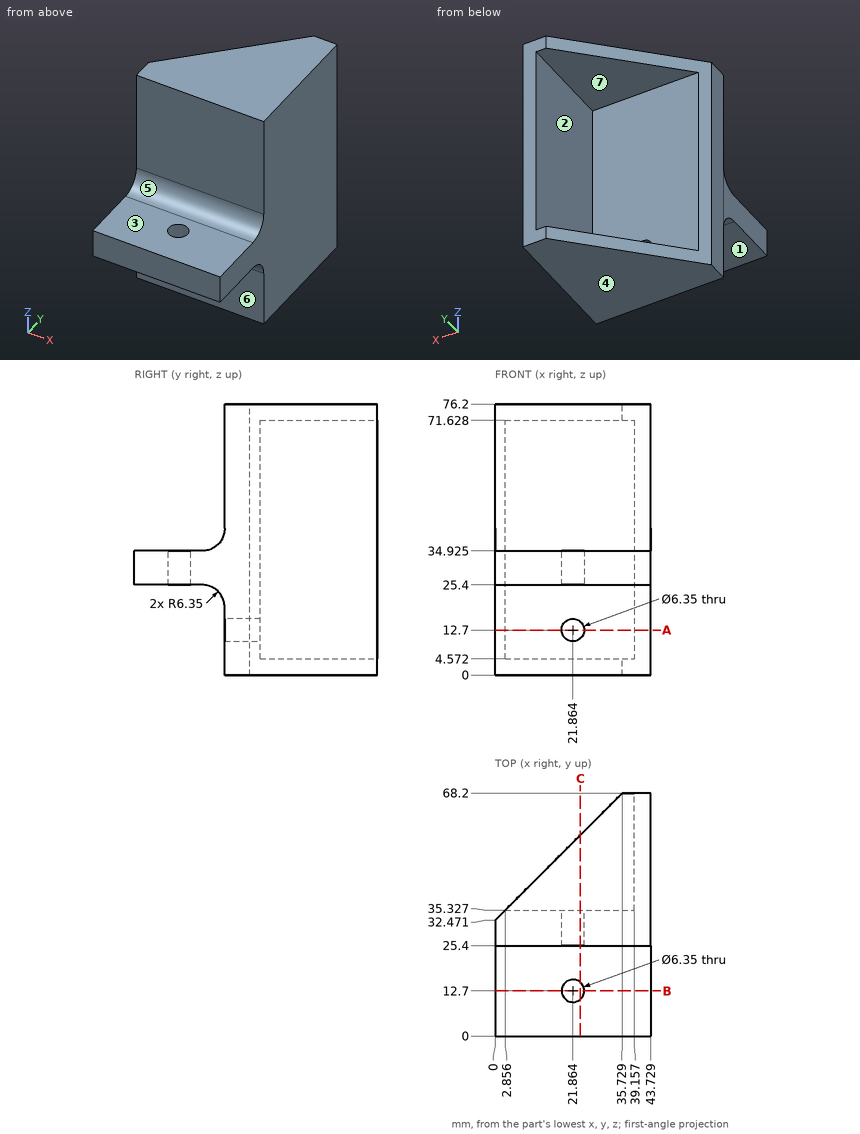
Geometry check sheet. Reference: drawing and pictorial views, mm from the part's lowest x, y, z. A direction names the side the tool comes from. Coordinates: 2 decimals unless noted, no trailing zeros. Order: outer loops, then holes, each group sorted by start corner. A loop starts at its lowest first (then second) coordinate and runs counter-clockwise, first axis right, second up.
Item 1: Tool access check on the marked faces 1, 2 and 3. Record the directions out of +Z, -Z, +X, -X, +Y, -Y that give a thin tool (end or side, any length) a straight path to the whole face; none if there is none.
Item 2: Section check A-A (z = 12.7). Enter the section's corners in (x, y).
Item 3: Depth check by flat-ended pin: pin 1 (17.5 mm diameter, centred on x = 32.5, z = 63, fed in from -Y); pin 2 (21 mm diameter, centred on x = 11, y = 10, fed in from -Z); pin 3 (5 mm diameter, centred on x = 29.5, z = 34, fed in from +Y). Enter the tip coordinate at first touch or a pass-through.
Item 4: Mould release check, pull along Z, two halves, no side actions. Record for the marked faces 4, 5, 6 and 7: released by +Z, released by -Z, zero draft, split by the parting line, or undercut.
Item 5: Scan lines: line 1 along Z through (x, y) = (17.5, 16) (1 decimal); line 2 along Y through (x, z) = (14, 19); line 3 along X through (y, z) = (12, 31). Record each from-to range of solid material in increasing order.
Item 6: Section check B-B (y = 12.7). Enter the section's corners in (x, z) (1 decimal).
Item 7: Section check C-C (x = 24). Count the separate pieces of the cut face and the enclosed holes in it, plus the area to 3 significant figures.
Check sheet entries:
1. face 1: -Z, +X, -X, -Y
1. face 2: -X, +Y
1. face 3: +Z, +X, -X, -Y
2. outline: (0, 25.4) - (18.69, 25.4) - (18.69, 35.33) - (2.86, 35.33) - (0, 32.47) - close; (25.04, 25.4) - (43.73, 25.4) - (43.73, 68.2) - (39.16, 68.2) - (39.16, 35.33) - (25.04, 35.33) - close
3. pin 1: stops at y = 25.4
3. pin 2: stops at z = 25.23
3. pin 3: stops at y = 35.33
4. face 4: released by -Z
4. face 5: released by +Z
4. face 6: zero draft
4. face 7: undercut
5. line 1: z = 25.4 to 34.9
5. line 2: y = 25.4 to 35.33
5. line 3: x = 0 to 18.77, 24.96 to 43.73
6. outline: (0, 25.4) - (18.7, 25.4) - (18.7, 34.9) - (0, 34.9) - close; (25, 25.4) - (43.7, 25.4) - (43.7, 34.9) - (25, 34.9) - close
7. separate pieces: 3
7. enclosed holes: 0
7. area: 1,120 mm2
